```python
from build123d import *

# Parameters (mm, degrees)
F1_DEPTH = 50.8
F2_W     = 8.733455
F2_H     = 13.649156
F3_DEPTH = 76.2


with BuildPart() as f1:
    # F0 (on Top) → F1 (new body)
    with BuildSketch(Plane.XY):
        Polygon((0, 50.8), (0, 0), (177.8, 0), align=None)
    extrude(amount=F1_DEPTH)

    # F2 (on face) → F3 (join)
    with BuildSketch(Plane.XY.offset(50.8)):
        Polygon((11.064442, 34.938731), (11.064442, 47.638731), (0, 50.8), (0, 0), (11.064442, 0), (11.064442, 9.0678), (23.764442, 9.0678), (23.764442, 0), (31.091255, 0), (31.091255, 41.916784), (23.764442, 44.010159), (23.764442, 34.938731), align=None)
        Polygon((58.754327, 34.01305), (40.974327, 39.09305), (40.974327, 0), (58.754327, 0), align=None)
        with Locations((50.614247, 15.892378)):
            Rectangle(F2_W, F2_H, mode=Mode.SUBTRACT)
        Polygon((80.572039, 27.779417), (69.328356, 30.991898), (69.328356, 0), (80.572039, 0), (85.649624, 6.265562), (88.696182, 15.811432), align=None)
        Polygon((75.697549, 9.908289), (75.697549, 15.495949), (75.697549, 19.873505), (80.572039, 15.923239), align=None, mode=Mode.SUBTRACT)
        Polygon((115.295707, 17.639365), (99.104117, 22.484538), (94.17998, 17.639365), (94.17998, 9.908289), (94.17998, 6.67177), (99.663779, 0), (107.178614, 0), (115.295707, 6.67177), (115.295707, 15.608329), align=None)
        Polygon((102.304123, 9.908289), (102.304123, 12.764879), (102.304123, 15.608329), (108.600341, 15.608329), (108.600341, 9.908289), align=None, mode=Mode.SUBTRACT)
    extrude(amount=-F3_DEPTH)


solid = f1.part
```
The listing builds one solid part. Answer for the finished solid, in the listing's coordinates (mm). A direction names the side the tool comes from. Coordinates: 2 decimals unless noted, no trailing zeros. Loops run counter-clockwise (first coordinate to the right, second up) from the corner with the lowest first, then second, coordinate; pieces in that order, holes last. Notation, with made-up numbers: (-25, 22) - (16, 22) arc R22 ccw to (16, 44) - close; hole circle Ø10 at (-1.5, 33). An arc over 180 degrees is marked (long way). Use a Markdown table: item, result. Add a question column.
1) For faces 1 (the flat face through (107.31, 20.03, -12.52)), 2 (the flat face through (11.064, 4, -13)), 3 (the flat face through (51, 16, 0)), 4 (the flat face through (11.064, 41, -13)), determine the directions among +Z, -Z, +X, -X, +Y, -Y from which every point of the face is accessible in a straight line to the end or side of a thin tool.
2) The part is cut by section B-B, the plane z = -18.5. State how many separate pieces and enclosed holes the cut face has, and give its area (3 significant figures).
3) The part is cut by section D-D, the plane x = 150. Give the vertices of the cut face in (y, z), and give its area (3 significant figures).
4) The part is cut by section A-A, the plane z = 45. Give the vertices of the cut face in (x, y), and give its area (3 significant figures).
5) The mould has two halves that part along X. Classify faces 5 (the flat face through (46, 20, -25.4)), 6 (the flat face through (78, 15, 0)), 7 (the flat face through (0, 26, 12)): released by +X, released by -X, zero draft, split by the parting line, or undercut.
6) Find the intervals of material crossed by line 1 (X direction, y = 27.5, z = -5); line 2 (X direction, y = 25.5, z = -19); line 3 (X direction, y = 33, z = -3), in increasing order.
7) Given pin 1 (2 mm diameter, centred on x = 148, z = 35, fed in from +Y); pin 2 (4.5 mm diameter, centred on x = 18.5, y = 2.5, fed in from -Z); pin 3 (5 mm diameter, centred on x = 107, z = -16, fed in from +Y), each flat-ended and moving along its own axis, determine where each tip first touches the part or whether it passes through.
Here are the results:
| question | item | result |
|---|---|---|
| 1 | face 1 | -Z, +X, +Y |
| 1 | face 2 | -Z, -Y |
| 1 | face 3 | -Z |
| 1 | face 4 | -Z, +Y |
| 2 | separate pieces | 4 |
| 2 | enclosed holes | 3 |
| 2 | area | 2,490 mm^2 |
| 3 | outline | (0, 0) - (7.94, 0) - (7.94, 50.8) - (0, 50.8) - close |
| 3 | area | 403 mm^2 |
| 4 | outline | (0, 0) - (177.8, 0) - (0, 50.8) - close |
| 4 | area | 4,520 mm^2 |
| 5 | face 5 | zero draft |
| 5 | face 6 | undercut |
| 5 | face 7 | released by -X |
| 6 | line 1 | x = 0 to 31.09, 40.97 to 58.75, 69.33 to 80.76 |
| 6 | line 2 | x = 0 to 31.09, 40.97 to 58.75, 69.33 to 82.12 |
| 6 | line 3 | x = 0 to 31.09, 40.97 to 58.75 |
| 7 | pin 1 | stops at y = 8.8 |
| 7 | pin 2 | stops at z = 0 |
| 7 | pin 3 | stops at y = 20.87 |
